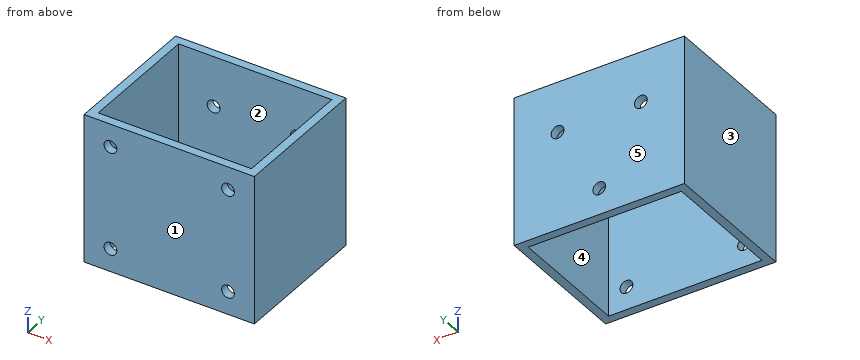
from build123d import *

# Parameters (mm, degrees)
SKETCH1_W           = 40
SKETCH1_H           = 33
SKETCH1_W_2         = 36
SKETCH1_H_2         = 29
BOSS_EXTRUDE1_DEPTH = 35
SKETCH2_R           = 1.5
CUT_EXTRUDE1_DEPTH  = 15
SKETCH3_R           = 1.5
CUT_EXTRUDE2_DEPTH  = 15


with BuildPart() as part:
    # Sketch1 → Boss-Extrude1 (new body)
    with BuildSketch(Plane.XY):
        Rectangle(SKETCH1_W, SKETCH1_H)
        Rectangle(SKETCH1_W_2, SKETCH1_H_2, mode=Mode.SUBTRACT)
    extrude(amount=BOSS_EXTRUDE1_DEPTH)

    # Sketch2 → Cut-Extrude1 (cut)
    with BuildSketch(Plane(origin=(0, 16.5, 0), x_dir=(1, 0, 0), z_dir=(0, 1, 0))):
        with Locations(Location((0, -6.2, 0), (0, 0, 180))):
            Circle(SKETCH2_R)
        with Locations(Location((9.786087063, -23.15, 0), (0, 0, 180))):
            Circle(SKETCH2_R)
        with Locations(Location((-9.786087063, -23.15, 0), (0, 0, 180))):
            Circle(SKETCH2_R)
    extrude(amount=-CUT_EXTRUDE1_DEPTH, mode=Mode.SUBTRACT)

    # Sketch3 → Cut-Extrude2 (cut)
    with BuildSketch(Plane.XZ.offset(16.5)):
        with Locations((13.809468579, 29.583285006)):
            Circle(SKETCH3_R)
        with Locations((-13.809468579, 29.583285006)):
            Circle(SKETCH3_R)
        with Locations(Location((13.809468579, 5.416714994, 0), (0, 0, 180))):
            Circle(SKETCH3_R)
        with Locations(Location((-13.809468579, 5.416714994, 0), (0, 0, 180))):
            Circle(SKETCH3_R)
    extrude(amount=-CUT_EXTRUDE2_DEPTH, mode=Mode.SUBTRACT)


solid = part.part
Read the model definition and answer for the solid it produces. Units are mm, in the model's axes. Face numbers are marked on the shaded views. A direction names the side the tool comes from. Give positions to 0.01 mm unless a question says otherwise; leave off trailing zeros. Write each loop counter-clockwise with the first axis right and the second up, starting at its lowest first coordinate (ties: lowest second). Pieces come first, ordered by that corner, then holes. Notation, with made-up numbers: M -4.5,13.5 L -0.5,13.5 A11 ccw -0.5,17.5 Z; hole C -27,17.25 d7. An arc over 180 degrees is marked long. One line per item, written item: value. Start each with the question number.
(1) A tool of negligible diameter and unlimited length cuts with its end or side. For the marked faces 1 and 2, from which of +Z, -Z, +X, -X, +Y, -Y can it reach the whole face along a straight path? Write none if from no direction.
(2) Find the intervals of material crossed by line 1 (X direction, y = 14, z = 5); line 2 (Y direction, x = 9.5, z = 8); line 3 (Y direction, x = -11, z = 23), in increasing order.
(3) Find section D-D (z = 2). Determine the outline of the cut face in (x, y), plus the area to 3 significant figures.
(4) Find section C-C (y = 3). Determine the outline of the cut face in (x, z), plus the area to 3 significant figures.
(5) Determine the mould class of the marked faces 3, 4 and 5 for opening direction Y: pulls with the +Y half, pulls with the -Y half, needs draft (parallel to the pull), parting line crosses it, or undercut.
(6) A flat-ended cylindrical pin translates along its axis: pin 1 Ø2.5 at (x, z) = (0, 6.2) entering from +Y. Find the tip coordinate at first contact, or state that the pin passes through.
(7) Find section B-B (x = 0). Determine the outline of the cut face in (y, z).
(8) Find section A-A (z = 23.15). Determine the outline of the cut face in (x, y), plus the area to 3 significant figures.
Results below:
1. face 1: +Z, -Z, +X, -X, -Y
1. face 2: +Z, -Z
2. line 1: x = -20 to -18, 18 to 20
2. line 2: y = -16.5 to -14.5, 14.5 to 16.5
2. line 3: y = -16.5 to -14.5
3. outline: M -20,-16.5 L 20,-16.5 L 20,16.5 L -20,16.5 Z; hole M -18,-14.5 L 18,-14.5 L 18,14.5 L -18,14.5 Z
3. area: 276 mm^2
4. outline: M -20,0 L -18,0 L -18,35 L -20,35 Z; M 18,0 L 20,0 L 20,35 L 18,35 Z
4. area: 140 mm^2
5. face 3: needs draft
5. face 4: undercut
5. face 5: pulls with the +Y half
6. pin 1: stops at y = -14.5
7. outline: M -16.5,0 L -14.5,0 L -14.5,35 L -16.5,35 Z; M 14.5,0 L 16.5,0 L 16.5,4.7 L 14.5,4.7 Z; M 14.5,7.7 L 16.5,7.7 L 16.5,35 L 14.5,35 Z
8. outline: M -20,-16.5 L 20,-16.5 L 20,16.5 L 11.29,16.5 L 11.29,14.5 L 18,14.5 L 18,-14.5 L -18,-14.5 L -18,14.5 L -11.29,14.5 L -11.29,16.5 L -20,16.5 Z; M -8.29,14.5 L 8.29,14.5 L 8.29,16.5 L -8.29,16.5 Z
8. area: 264 mm^2
